Geometry check sheet. Reference: the model listing, model coordinates, mm. Round coordinates to 2 decimals unless told otherwise and drop trailing zeros. Write each loop counter-clockwise with the first axis right and the second up, starting at its lowest first coordinate (ties: lowest second). Pieces come first, ordered by that corner, then holes.
Item 1: Cross-section at A-A (z = 9). Enter the section's corners in (x, y), then the cut area to 3 significant figures.
Item 2: Scan lines: probe 1 along X at (y, z) = (79, 5.75); probe 2 along Y at (x, z) = (135, 7.5); probe 3 along X at (y, z) = (27.5, 7.25). Record each from-to range of solid material in increasing order.
Item 3: Depth check by flat-ended pin: P1, Ø6, axis at y = 26, z = 13, coming from the -X side; P2, Ø3, axis at y = 10, z = 15, coming from the +X side; P3, Ø5, axis at x = 201.5, z = 13, coming from the -Y side; P4, Ø6, axis at x = 193.5, y = 37.5, coming from the -Z side. Enter the tip coordinate at first touch or a pass-through.
Item 4: Cross-section at B-B (x = 132.5). Enter the section's corners in (y, z).
from build123d import *

# Parameters (mm, degrees)
F2_DEPTH = 25.4
F3_R     = 25.39999


# Not quite as in the source:
# - a fillet or chamfer is up to 0.001 mm smaller than in the source, because OpenCascade refuses the exact size


with BuildPart() as f2:
    # F1 (on face) → F2 (new body)
    with BuildSketch(Plane.XY):
        with BuildLine():
            Line((210.4652929995, 89.2318353651), (121.2334576344, 0))
            Line((121.2334576344, 0), (161.6446101792, 0))
            Line((161.6446101792, 0), (220.8106438897, 59.1660337104))
            ThreePointArc((220.8106438897, 59.1660337104), (216.1613322086, 74.3790189354), (210.4652929995, 89.2318353651))
        make_face()
    extrude(amount=F2_DEPTH)

    # F3 (radius 25.4 in the source; OpenCascade refuses exactly that, so slightly less here)
    f3_edges = [f2.edges().sort_by_distance(p)[0] for p in [
        (216.161332, 74.379019, 25.4),
    ]]
    fillet(f3_edges, radius=F3_R)


solid = f2.part
Resolved:
1. outline: (121.23, 0) - (161.64, 0) - (219.46, 57.82) arc R226.95 ccw to (209.21, 87.97) - close
1. area: 2,960 mm2
2. probe 1: x = 200.23 to 213.81
2. probe 2: y = 0 to 13.77
2. probe 3: x = 148.73 to 189.14
3. P1: stops at x = 144.23
3. P2: stops at x = 173.14
3. P3: stops at y = 37.36
3. P4: stops at z = 0
4. outline: (0, 0) - (11.27, 0) - (11.27, 25.4) - (0, 25.4) - close
